from build123d import *

# Parameters (mm, degrees)
BOSS_EXTRUDE1_DEPTH = 2


with BuildPart() as part:
    # Sketch2 → Boss-Extrude1 (new body)
    with BuildSketch(Plane.XY):
        with BuildLine():
            Line((38, 0), (-38, 0))
            Line((-38, 0), (-38, -67))
            Line((-38, -67), (-40, -67))
            Line((-40, -67), (-40, -71))
            ThreePointArc((-40, -71), (0, -76.708339656), (40, -71))
            Line((40, -71), (40, -67))
            Line((40, -67), (38, -67))
            Line((38, -67), (38, 0))
        make_face()
    extrude(amount=BOSS_EXTRUDE1_DEPTH)


solid = part.part
CAD build for the part. Positions are in the model's coordinates, mm. A direction names the side the tool comes from. Give positions to 0.01 mm unless a question says otherwise; leave off trailing zeros. Loops run counter-clockwise (first coordinate to the right, second up) from the corner with the lowest first, then second, coordinate; pieces in that order, holes last. Notation, with made-up numbers: M -5.5,35 L 10.5,35 A23 ccw 10.5,55 Z; hole C 49.5,-14 d9. An arc over 180 degrees is marked long. One line per question, with ' | ' between items. Start each with the question number.
1. Saw through at A-A on z = 1.1. Give the cut face in (x, y), plus the area to 3 significant figures.
2. Saw through at B-B on y = -46. Give the cut face in (x, z), plus the area to 3 significant figures.
3. 3-axis set-ups, long thin cutter, end or side, ignore diameter. For faces 1 (the face through (38, -34, 1)), 2 (the face through (1, 0, 1)), 3 (the face through (-39, -67, 1)): which of +Z, -Z, +X, -X, +Y, -Y reach the whole face in a straight line?
4. Flat gauge pins, fed straight in: pin 1 (1 mm diameter, centred on x = -39, z = 1, fed in from +Y); pin 2 (1 mm diameter, centred on y = -18, z = 0.5, fed in from -X). Where does each tip first touch, or does it go through?
5. Saw through at C-C on x = -31. Give the cut face in (y, z).
6. Two-plate mould, pull along X, no slides. Class faces 4 (the face through (-40, -69, 1)), 5 (the face through (-1, -38, 2)), 6 (the face through (-0.568, -76.707, 0.986)), 7 (the face through (40, -69, 1)): pulls with the +X half, pulls with the -X half, needs draft (parallel to the pull), parting line crosses it, or undercut.
7. Probe L1, parallel to X at y = -4.5, z = 0.75; L2, parallel to Y at x = 22, z = 1.3; L3, parallel to Y at x = 14, z = 0.55. List the from-to ranges inside material, lowest first. Write a range as from..to.
Result sheet:
1) outline: M -40,-71 A143 ccw 40,-71 L 40,-67 L 38,-67 L 38,0 L -38,0 L -38,-67 L -40,-67 Z | area: 5,720 mm^2
2) outline: M -38,0 L 38,0 L 38,2 L -38,2 Z | area: 152 mm^2
3) face 1: +Z, -Z, +X, +Y | face 2: +Z, -Z, +X, -X, +Y | face 3: +Z, -Z, -X, +Y
4) pin 1: stops at y = -67 | pin 2: stops at x = -38
5) outline: M -73.31,0 L 0,0 L 0,2 L -73.31,2 Z
6) face 4: pulls with the -X half | face 5: needs draft | face 6: parting line crosses it | face 7: pulls with the +X half
7) L1: x = -38..38 | L2: y = -75.01..0 | L3: y = -76.02..0
